Geometry check sheet. Reference: the model listing, model coordinates, mm. Face numbers are marked on the shaded views. Coordinates: 2 decimals unless noted, no trailing zeros. Write each loop counter-clockwise with the first axis right and the second up, starting at its lowest first coordinate (ties: lowest second). Pieces come first, ordered by that corner, then holes. Notation, with made-up numbers: M -1.75,32 L 11.25,32 A28 ccw 11.25,71 Z; hole C 34,60.5 d1. An arc over 180 degrees is marked long. Write each question's results on one line, items separated by ' | '.
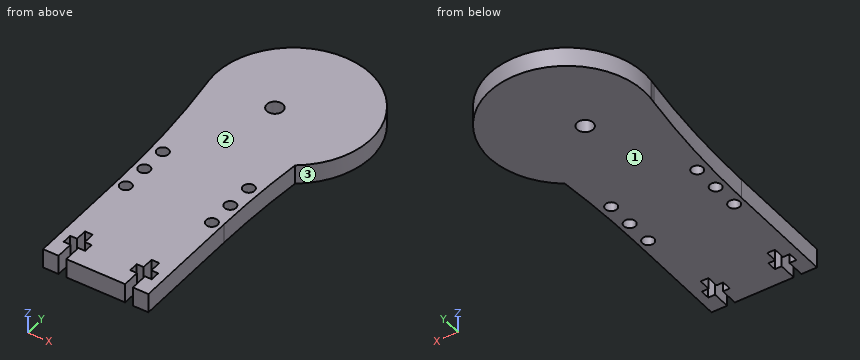
```python
from build123d import *

# Parameters (mm, degrees)
RESSALTO_EXTRUS_O1_DEPTH = 5
ESBO_O7_R                = 2.076684074
CORTE_EXTRUS_O5_DEPTH    = 6
ESBO_O8_W                = 32.941442616
ESBO_O8_H                = 7.70353162
CORTE_EXTRUS_O6_DEPTH    = 6
ESBO_O9_R                = 1.5
CORTE_EXTRUS_O7_DEPTH    = 6
ESBO_O10_W               = 2
ESBO_O10_H               = 3
CORTE_EXTRUS_O8_DEPTH    = 6


with BuildPart() as part:
    # Esboço1 → Ressalto-extrusão1 (new body)
    with BuildSketch(Plane.XY):
        with BuildLine():
            Line((13.569146061, 27.715579822), (13.569146061, 56.338894978))
            ThreePointArc((13.569146061, 56.338894978), (13.884544414, 68.892766914), (14.829943665, 81.414963086))
            ThreePointArc((14.829943665, 81.414963086), (11.193742071, 116.066691762), (-16.576524471, 95.024435265))
            Line((-16.576524471, 95.024435265), (-16.487894969, 94.437265709))
            Line((-16.487894969, 94.437265709), (-16.369382775, 93.652123615))
            ThreePointArc((-16.369382775, 93.652123615), (-14.270188159, 75.047972701), (-13.569146061, 56.338894978))
            Line((-13.569146061, 56.338894978), (-13.569146061, 27.715579822))
            ThreePointArc((-13.569146061, 27.715579822), (0, 21.02683783), (13.569146061, 27.715579822))
        make_face()
    extrude(amount=RESSALTO_EXTRUS_O1_DEPTH)

    # Esboço7 → Corte-extrusão5 (cut, through all)
    with BuildSketch(Plane(origin=(0, 0, 0), x_dir=(-1, 0, 0), z_dir=(0, 0, -1))):
        with Locations((-0.267564972, 95.19)):
            Circle(ESBO_O7_R)
    extrude(amount=-CORTE_EXTRUS_O5_DEPTH, mode=Mode.SUBTRACT)

    # Esboço8 → Corte-extrusão6 (cut, through all)
    with BuildSketch(Plane.XY.offset(5)):
        with Locations((-2.901575247, 23.863814012)):
            Rectangle(ESBO_O8_W, ESBO_O8_H)
    extrude(amount=-CORTE_EXTRUS_O6_DEPTH, mode=Mode.SUBTRACT)

    # Esboço9 → Corte-extrusão7 (cut, through all)
    with BuildSketch(Plane(origin=(0, 0, 0), x_dir=(-1, 0, 0), z_dir=(0, 0, -1))):
        with Locations((11.072435028, 69.41)):
            Circle(ESBO_O9_R)
        with Locations((11.072435028, 62.41)):
            Circle(ESBO_O9_R)
        with Locations((11.072435028, 55.41)):
            Circle(ESBO_O9_R)
        with Locations((-11.067564972, 69.41)):
            Circle(ESBO_O9_R)
        with Locations((-11.067564972, 62.41)):
            Circle(ESBO_O9_R)
        with Locations((-11.067564972, 55.41)):
            Circle(ESBO_O9_R)
    extrude(amount=-CORTE_EXTRUS_O7_DEPTH, mode=Mode.SUBTRACT)

    # Esboço10 → Corte-extrusão8 (cut, through all)
    with BuildSketch(Plane(origin=(0, 0, 0), x_dir=(-1, 0, 0), z_dir=(0, 0, -1))):
        Polygon((7.569146061, 27.715579822), (9.569146061, 27.715579822), (9.569146061, 32.265579822), (11.339146061, 32.265579822), (11.339146061, 34.715579822), (9.569146061, 34.715579822), (7.569146061, 34.715579822), (5.799146061, 34.715579822), (5.799146061, 32.265579822), (7.569146061, 32.265579822), align=None)
        with Locations((8.569146061, 36.215579822)):
            Rectangle(ESBO_O10_W, ESBO_O10_H)
        Polygon((-9.569146061, 27.715579822), (-7.569146061, 27.715579822), (-7.569146061, 32.265579822), (-5.799146061, 32.265579822), (-5.799146061, 34.715579822), (-7.569146061, 34.715579822), (-7.569146061, 37.715579822), (-9.569146061, 37.715579822), (-9.569146061, 34.715579822), (-11.339146061, 34.715579822), (-11.339146061, 32.265579822), (-9.569146061, 32.265579822), align=None)
    extrude(amount=-CORTE_EXTRUS_O8_DEPTH, mode=Mode.SUBTRACT)


solid = part.part
```
Q1. Sectioned sample at B-B on y = 69.41. Record the cut outline in (x, z).
Geometry check:
outline: M -13.91,0 L -12.57,0 L -12.57,5 L -13.91,5 Z; M -9.57,0 L 9.57,0 L 9.57,5 L -9.57,5 Z; M 12.57,0 L 13.91,0 L 13.91,5 L 12.57,5 Z
Q2. Sectioned sample at D-D on x = -8.5. Record the cut outline in (y, z), and give its area (3 significant figures).
Geometry check:
outline: M 37.72,0 L 113.91,0 L 113.91,5 L 37.72,5 Z | area: 381 mm2
Q3. Sectioned sample at A-A on y = 55.41. Record the cut outline in (x, z).
Geometry check:
outline: M -13.57,0 L -12.57,0 L -12.57,5 L -13.57,5 Z; M -9.57,0 L 9.57,0 L 9.57,5 L -9.57,5 Z; M 12.57,0 L 13.57,0 L 13.57,5 L 12.57,5 Z
Q4. Depth check by flat-ended pin: P1, Ø2.5, axis at y = 34, z = 3.5, coming from the -X side; P2, Ø2.5, axis at x = -11.07, y = 69.41, coming from the -Z side; P3, Ø3, axis at x = -0.5, z = 2.5, coming from the +Y side; P4, Ø3, axis at y = 44.5, z = 2.5, coming from the +X side. Enter the tip coordinate at first touch or a pass-through.
Geometry check:
P1: stops at x = -13.57 | P2: passes through | P3: stops at y = 117.59 | P4: stops at x = 13.57
Q5. Mould release check, pull along Z, two halves, no side actions. Record for the marked faces 1, 2 and 3: pulls with the +Z half, pulls with the -Z half, needs draft (parallel to the pull), parting line crosses it, or undercut.
Geometry check:
face 1: pulls with the -Z half | face 2: pulls with the +Z half | face 3: needs draft
Q6. Scan lines: probe 1 along X at (y, z) = (69.41, 3.8); probe 2 along Y at (x, z) = (10.5, 0.85); probe 3 along Y at (x, z) = (4, 3.9). Record each from-to range of solid material in increasing order.
Geometry check:
probe 1: x = -13.91 to -12.57, -9.57 to 9.57, 12.57 to 13.91 | probe 2: y = 27.72 to 32.27, 34.72 to 54.02, 56.8 to 61.02, 63.8 to 68.02, 70.8 to 116.35 | probe 3: y = 27.72 to 117.7
Q7. Sectioned sample at C-C on z = 3.15. Give the number of separate pieces and of enclosed holes in the cut face, and give its area (3 significant figures).
Geometry check:
separate pieces: 1 | enclosed holes: 7 | area: 2,590 mm2
